Build history of the part. All positions in model axes, mm. A direction names the side the tool comes from. Coordinates: 2 decimals unless noted, no trailing zeros. Loops run counter-clockwise (first coordinate to the right, second up) from the corner with the lowest first, then second, coordinate; pieces in that order, holes last. Notation, with made-up numbers: (-1.5, -10) - (19.5, -10) arc R24 ccw to (19.5, 26) - close; hole circle Ø9 at (61, -32.75). An arc over 180 degrees is marked (long way). One line per item, written item: value.
```python
from build123d import *

# Parameters (mm, degrees)
SKETCH_1_R                     = 36
EXTRUDE_1_DEPTH                = 4
SKETCH_2_R                     = 22.5
EXTRUDE_2_DEPTH                = 6
SKETCH_3_R                     = 12.5
EXTRUDE_3_DEPTH                = 3
SKETCH_4_R                     = 8.5
EXTRUDE_4_DEPTH                = 64
SKETCH_5_R                     = 8.1
EXTRUDE_5_DEPTH                = 1.1
SKETCH_6_R                     = 8.5
EXTRUDE_6_DEPTH                = 3.9
CHAMFER_1_SIZE                 = 1
HOLE_WIZARD_6_0_6_1_AT_2_COUNT = 2
HOLE_WIZARD_6_0_6_1_AT_2_PITCH = 51.961524227
HOLE_WIZARD_6_0_6_1_AT_3_COUNT = 2
HOLE_WIZARD_6_0_6_1_AT_3_PITCH = 51.961524227
CUT_EXTRUDE_START              = -5.5
CUT_EXTRUDE_1_DEPTH            = 92.019428096


with BuildPart() as part:
    # 草图1 → 凸台-拉伸1 (new body)
    with BuildSketch(Plane.XY):
        Circle(SKETCH_1_R)
    extrude(amount=EXTRUDE_1_DEPTH)

    # 草图2 → 凸台-拉伸2 (add)
    with BuildSketch(Plane.XY.offset(4)):
        Circle(SKETCH_2_R)
    extrude(amount=EXTRUDE_2_DEPTH)

    # 草图3 → 凸台-拉伸3 (add)
    with BuildSketch(Plane.XY.offset(10)):
        Circle(SKETCH_3_R)
    extrude(amount=EXTRUDE_3_DEPTH)

    # 草图4 → 凸台-拉伸4 (add)
    with BuildSketch(Plane.XY.offset(13)):
        Circle(SKETCH_4_R)
    extrude(amount=EXTRUDE_4_DEPTH)

    # 草图5 → 凸台-拉伸5 (add)
    with BuildSketch(Plane.XY.offset(77)):
        Circle(SKETCH_5_R)
    extrude(amount=EXTRUDE_5_DEPTH)

    # 草图6 → 凸台-拉伸6 (add)
    with BuildSketch(Plane.XY.offset(78.1)):
        Circle(SKETCH_6_R)
    extrude(amount=EXTRUDE_6_DEPTH)

    # 倒角1
    chamfer_1_edges = [part.edges().sort_by_distance(p)[0] for p in [
        (-8.5, 0, 82),
    ]]
    chamfer(chamfer_1_edges, length=CHAMFER_1_SIZE)

    # 草图8 → Ø6.0 (6) 直径孔1 (revolve, cut)
    with BuildSketch(Plane(origin=(-25.980762114, -15, 0), x_dir=(0, 1, 0), z_dir=(1, 0, 0))):
        Polygon((0, 0), (0, 4), (3, 4), (3, 2.5), (5.5, 0), align=None)
    hole_wizard_6_0_6_1 = revolve(axis=Axis((-25.980762114, -15, -6.35), (0, 0, 1)), mode=Mode.SUBTRACT)

    # Ø6.0 (6) 直径孔1 at 2: Ø6.0 (6) 直径孔1 ×2
    with Locations(*[Vector(0.499999999999998, 0.8660254037844398, 0) * (i * HOLE_WIZARD_6_0_6_1_AT_2_PITCH) for i in range(1, HOLE_WIZARD_6_0_6_1_AT_2_COUNT)]):
        add(hole_wizard_6_0_6_1, mode=Mode.SUBTRACT)

    # Ø6.0 (6) 直径孔1 at 3: Ø6.0 (6) 直径孔1 ×2
    with Locations(*[(i * HOLE_WIZARD_6_0_6_1_AT_3_PITCH, 0, 0) for i in range(1, HOLE_WIZARD_6_0_6_1_AT_3_COUNT)]):
        add(hole_wizard_6_0_6_1, mode=Mode.SUBTRACT)

    # 草图9 → 切除-拉伸1 (cut, through all)
    with BuildSketch(Plane(origin=(0, 0, 0), x_dir=(0, 0, -1), z_dir=(1, 0, 0)).offset(CUT_EXTRUDE_START)):
        with BuildLine():
            Line((-72.5, 2.5), (-57.5, 2.5))
            ThreePointArc((-57.5, 2.5), (-55, 0), (-57.5, -2.5))
            Line((-57.5, -2.5), (-72.5, -2.5))
            ThreePointArc((-72.5, -2.5), (-75, 0), (-72.5, 2.5))
        make_face()
    extrude(amount=-CUT_EXTRUDE_1_DEPTH, mode=Mode.SUBTRACT)


solid = part.part
```
Item 1: Cut at B-B, the plane y = 30. Write the cut outline in (x, z).
Check result:
outline: (-19.9, 0) - (-5.5, 0) - (-3, 2.5) - (-3, 4) - (-19.9, 4) - close; (3, 2.5) - (5.5, 0) - (19.9, 0) - (19.9, 4) - (3, 4) - close
Item 2: Probe probe 1 along X at (y, z) = (-15, 3.3); probe 2 along Y at (x, z) = (0, 3.6); probe 3 along Z at (x, y) = (27, -1). List the from-to ranges inside material, lowest first. Write a range as from..to.
Check result:
probe 1: x = -32.73..-28.98, -22.98..22.98, 28.98..32.73
probe 2: y = -36..27, 33..36
probe 3: z = 0..4
Item 3: Cut at D-D, the plane y = -15. Write the cut outline in (x, z).
Check result:
outline: (-32.73, 0) - (-31.48, 0) - (-28.98, 2.5) - (-28.98, 4) - (-32.73, 4) - close; (-22.98, 2.5) - (-20.48, 0) - (20.48, 0) - (22.98, 2.5) - (22.98, 4) - (16.77, 4) - (16.77, 10) - (-16.77, 10) - (-16.77, 4) - (-22.98, 4) - close; (28.98, 2.5) - (31.48, 0) - (32.73, 0) - (32.73, 4) - (28.98, 4) - close
Item 4: Drop flat-ended pins along their axis: P1, Ø1.3, axis at x = -7, z = 62, coming from the -Y side; P2, Ø5.5, axis at x = 0, y = 30, coming from the -Z side; P3, Ø5.5, axis at y = 0, z = 67, coming from the -X side; P4, Ø8, axis at x = 25.98, y = -15, coming from the +Z side. Give the stop position or say it passes through.
Check result:
P1: stops at y = -5.65
P2: passes through
P3: stops at x = -8.12
P4: stops at z = 4
Item 5: Tool access for faces 1 (the face through (-3, -8.2, 13)), 2 (the face through (-7, 0, 55)), 3 (the face through (-1.756, -7.907, 77.542)): list every direction of +Z, -Z, +X, -X, +Y, -Y with a clear straight run to the whole face (end or side of a thin tool).
Check result:
face 1: +Z
face 2: -X
face 3: none
Item 6: Pull direction Y, two halves, no side cores. Call faces 4 (the face through (-7, -2.5, 65)), 5 (the face through (0, 0, 82)), 6 (the face through (11.923, 3.755, 11.479)): released by +Y, released by -Y, zero draft, split by the parting line, or undercut.
Check result:
face 4: undercut
face 5: zero draft
face 6: split by the parting line
